For this review, take the finished solid that the model builds, in its own axes (mm). Face numbers are marked on the shaded views. A direction names the side the tool comes from. Give positions to 0.01 mm unless a question says otherwise; leave off trailing zeros. Write each loop counter-clockwise with the first axis right and the second up, starting at its lowest first coordinate (ties: lowest second). Pieces come first, ordered by that corner, then holes.
Q1. Insertion check: P1, Ø0.6, axis at x = 3, y = -10, coming from the +Z side; P2, Ø1, axis at x = 8.5, z = 2.5, coming from the +Y side. Each pin has a flat end and moves straight along its axis. Give the tip position at first contact, or say it passes through.
Q2. For line 1 (Z direction, x = 7, y = -7.5); line 2 (Z direction, x = 17, y = -15.25), list the stretches that pass through material, from the lowest coordinate up.
Q3. We need section B-B (x = 7). Write out the cut boundary in (y, z), then the cut area to 3 significant figures.
Q4. We need section A-A (z = 8.25). Give the number of separate pieces and of enclosed holes in the cut face, then the cut area to 3 significant figures.
Q5. Machinability: for the marked faces 4 and 5, which of the approach directions +Z, -Z, +X, -X, +Y, -Y give a long, thin tool a straight path to every point of the face, cutting with its end or side? Answer none if there is none.
Q6. Mouldability with a two-part tool opening along X and no side actions: class the marked faces 1, 2 and 3 as released by +X, released by -X, zero draft, split by the parting line, or undercut.
```python
from build123d import *

# Parameters (mm, degrees)
F0_W     = 31.242
F0_H     = 11.0998
F1_DEPTH = 27.3558
F2_W     = 3.468914
F2_H     = 9.1186
F2_W_2   = 3.468915
F3_DEPTH = 27.3568
F4_R     = 0.79375


with BuildPart() as f1:
    # F0 (on Front) → F1 (new body)
    with BuildSketch(Plane.XZ):
        with Locations((15.621, 5.5499)):
            Rectangle(F0_W, F0_H)
    extrude(amount=F1_DEPTH)

    # F2 (on face) → F3 (cut, through all)
    with BuildSketch(Plane.XZ.offset(27.3558)):
        with Locations((2.928257, 6.5405)):
            Rectangle(F2_W, F2_H)
        with Locations((7.159171, 6.5405)):
            Rectangle(F2_W_2, F2_H)
        with Locations((11.390086, 6.5405)):
            Rectangle(F2_W, F2_H)
        with Locations((15.621, 6.5405)):
            Rectangle(F2_W, F2_H)
        with Locations((19.851914, 6.5405)):
            Rectangle(F2_W, F2_H)
        with Locations((24.082828, 6.5405)):
            Rectangle(F2_W_2, F2_H)
        with Locations((28.313743, 6.5405)):
            Rectangle(F2_W, F2_H)
    extrude(amount=-F3_DEPTH, mode=Mode.SUBTRACT)

    # F4
    f4_edges = [f1.edges().sort_by_distance(p)[0] for p in [
        (1.1938, -13.6779, 1.9812),
        (4.662714, -13.6779, 1.9812),
        (5.424714, -13.6779, 1.9812),
        (8.893629, -13.6779, 1.9812),
        (9.655629, -13.6779, 1.9812),
        (13.124543, -13.6779, 1.9812),
        (13.886543, -13.6779, 1.9812),
        (17.355457, -13.6779, 1.9812),
        (18.117457, -13.6779, 1.9812),
        (21.586371, -13.6779, 1.9812),
        (22.348371, -13.6779, 1.9812),
        (25.817286, -13.6779, 1.9812),
        (26.579286, -13.6779, 1.9812),
        (30.0482, -13.6779, 1.9812),
    ]]
    fillet(f4_edges, radius=F4_R)


solid = f1.part
```
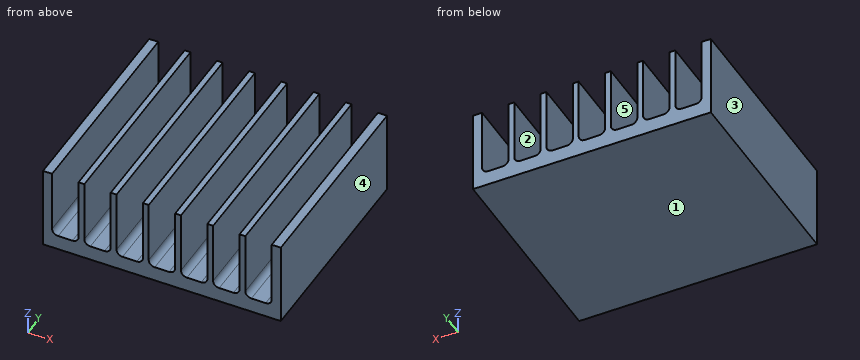
Computed:
1. P1: stops at z = 1.98
1. P2: stops at y = 0
2. line 1: z = 0 to 1.98
2. line 2: z = 0 to 2.11
3. outline: (-27.36, 0) - (0, 0) - (0, 1.98) - (-27.36, 1.98) - close
3. area: 54.2 mm2
4. separate pieces: 8
4. enclosed holes: 0
4. area: 190 mm2
5. face 4: +Z, -Z, +X, +Y, -Y
5. face 5: +Z, +Y, -Y
6. face 1: zero draft
6. face 2: undercut
6. face 3: released by -X
